Check sheet for the modelled part. Datum: model origin and axes. Units: mm. Face numbers are marked on the shaded views. A direction names the side the tool comes from. Give positions to 0.01 mm unless a question says otherwise; leave off trailing zeros. Order: outer loops, then holes, each group sorted by start corner. A loop starts at its lowest first (then second) coordinate and runs counter-clockwise, first axis right, second up.
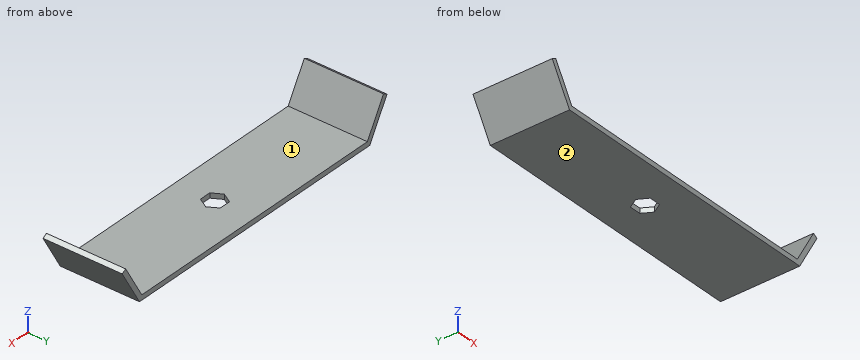
```python
from build123d import *

# Parameters (mm, degrees)
F0_W     = 177.8
F0_H     = 50.8
F1_DEPTH = 3.175
F3_DEPTH = 25.4


with BuildPart() as f1:
    # F0 (on Top) → F1 (new body)
    with BuildSketch(Plane.XY):
        Rectangle(F0_W, F0_H)
        Polygon((-3.666174, -6.35), (-7.332348, 0), (-3.666174, 6.35), (3.666174, 6.35), (7.332348, 0), (3.666174, -6.35), align=None, mode=Mode.SUBTRACT)
    extrude(amount=F1_DEPTH)

    # F2 (on Front) → F3 (join, symmetric)
    with BuildSketch(Plane.XZ):
        Polygon((-104.349631, 23.584545), (-90.733087, 0), (-88.9, 0), (-88.9, 3.175), (-101.6, 25.172045), align=None)
        Polygon((104.349631, 23.584545), (101.6, 25.172045), (88.9, 3.175), (88.9, 0), (90.733087, 0), align=None)
    extrude(amount=F3_DEPTH, both=True)


solid = f1.part
```
(1) Cross-section at D-D on x = -19.5. Enter the section's corners in (y, z) (3 decimals), then the cut area to 3 significant figures.
Response values:
outline: (-25.4, 0) - (25.4, 0) - (25.4, 3.175) - (-25.4, 3.175) - close
area: 161 mm2
(2) Cross-section at A-A on y = -3.5. Enter the section's corners in (x, z) (3 decimals), then the cut area to 3 significant figures.
Response values:
outline: (-104.35, 23.585) - (-90.733, 0) - (-5.312, 0) - (-5.312, 3.175) - (-88.9, 3.175) - (-101.6, 25.172) - close; (5.312, 0) - (90.733, 0) - (104.35, 23.585) - (101.6, 25.172) - (88.9, 3.175) - (5.312, 3.175) - close
area: 704 mm2
(3) Set-up check for the marked faces 1 and 2: record each of +Z, -Z, +X, -X, +Y, -Y from which the full face is reachable in a straight line by a thin tool's end or side.
Response values:
face 1: +Z, +Y, -Y
face 2: -Z, +X, -X, +Y, -Y
(4) Gauge pin test, flat ends, axial feed: pin 1 Ø15 at (x, y) = (25, 1) entering from +Z (3 decimals); pin 2 Ø10 at (y, z) = (-20.5, 11) entering from -X; pin 3 Ø5 at (y, z) = (-4, 21) entering from -X. Record the tip position at first contact, or that the pin passes through.
Response values:
pin 1: stops at z = 3.175
pin 2: stops at x = -99.97
pin 3: stops at x = -104.3
(5) Cross-section at C-C on y = 14.5. Enter the section's corners in (x, z) (3 decimals), then the cut area to 3 significant figures.
Response values:
outline: (-104.35, 23.585) - (-90.733, 0) - (90.733, 0) - (104.35, 23.585) - (101.6, 25.172) - (88.9, 3.175) - (-88.9, 3.175) - (-101.6, 25.172) - close
area: 737 mm2
(6) Material ranges on L1, parallel to Z at x = 66, y = 11 (3 decimals); L2, parallel to X at y = 17.5, z = 5; L3, parallel to X at y = 17.5, z = 22.25, recorded low to high.
Response values:
L1: z = 0 to 3.175
L2: x = -93.62 to -89.95, 89.95 to 93.62
L3: x = -103.58 to -99.91, 99.91 to 103.58
(7) Cross-section at B-B on z = 18.5. Enter the section's corners in (x, y), then the cut area to 3 significant figures.
Response values:
outline: (-101.41, -25.4) - (-97.75, -25.4) - (-97.75, 25.4) - (-101.41, 25.4) - close; (97.75, -25.4) - (101.41, -25.4) - (101.41, 25.4) - (97.75, 25.4) - close
area: 372 mm2
